Read the model definition and answer for the solid it produces. Units are mm, in the model's axes. Face numbers are marked on the shaded views. A direction names the side the tool comes from. Coordinates: 2 decimals unless noted, no trailing zeros. Loops run counter-clockwise (first coordinate to the right, second up) from the corner with the lowest first, then second, coordinate; pieces in that order, holes last.
from build123d import *

# Parameters (mm, degrees)
F1_DEPTH = 38.1
F2_R     = 3.175
F3_DEPTH = 25.4
F4_R     = 6.35
F6_DEPTH = 12.7
F7_R     = 12.7
F8_R     = 12.7


with BuildPart() as f1:
    # F0 (on Front) → F1 (new body)
    with BuildSketch(Plane.XZ):
        Polygon((19.5751538399, 3.9005766285), (19.3787731311, 22.9495643868), (-25.0712268689, 22.9495643868), (-25.0712268689, 18.1870643868), (-6.0212268689, 18.1870643868), (-6.0212268689, 8.6620643868), (-24.8748461601, 8.6620643868), (-24.8748461601, 3.9005766285), align=None)
    extrude(amount=-F1_DEPTH)

    # F2 (on face) → F3 (cut)
    with BuildSketch(Plane.XY.offset(22.9495643868)):
        with Locations((-15.5462268689, 28.575)):
            Circle(F2_R)
        with Locations((-15.5462268689, 9.525)):
            Circle(F2_R)
    extrude(amount=-F3_DEPTH, mode=Mode.SUBTRACT)

    # F4
    f4_edges = [f1.edges().sort_by_distance(p)[0] for p in [
        (-25.071227, 0, 20.568314),
        (-24.874846, 0, 6.281321),
        (-24.874846, 38.1, 6.281321),
        (-25.071227, 38.1, 20.568314),
    ]]
    fillet(f4_edges, radius=F4_R)

    # F5 (on face) → F6 (cut)
    with BuildSketch(Plane(origin=(19.613281335, 0, 0.2021981503), x_dir=(0, 1, 0), z_dir=(0.999946864, 0, 0.0103086986))):
        with BuildLine():
            Line((12.7, 13.2235750059), (25.4, 13.2235750059))
            ThreePointArc((25.4, 13.2235750059), (19.05, 19.5735750059), (12.7, 13.2235750059))
        make_face()
        with BuildLine():
            ThreePointArc((12.7, 13.2235750059), (19.05, 6.8735750059), (25.4, 13.2235750059))
            Line((25.4, 13.2235750059), (12.7, 13.2235750059))
        make_face()
    extrude(amount=-F6_DEPTH, mode=Mode.SUBTRACT)

    # F7
    f7_edges = [f1.edges().sort_by_distance(p)[0] for p in [
        (-6.021227, 0, 13.424564),
    ]]
    fillet(f7_edges, radius=F7_R)

    # F8
    f8_edges = [f1.edges().sort_by_distance(p)[0] for p in [
        (-6.021227, 38.1, 13.424564),
    ]]
    fillet(f8_edges, radius=F8_R)


solid = f1.part
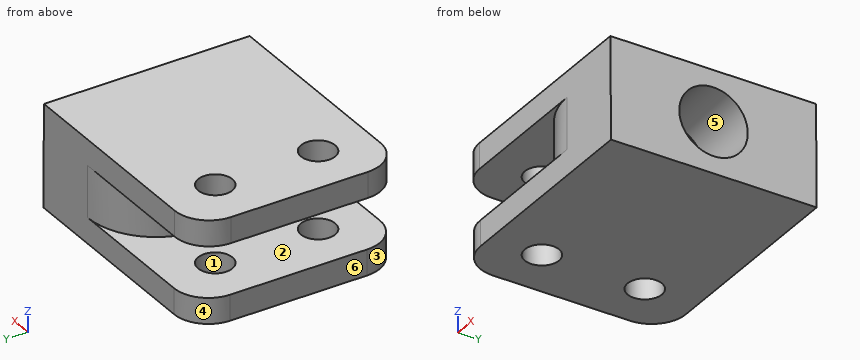
Item 1: A cutting plane is placed at A-A on x = -9. Determine the outline of the cut face in (y, z), then the cut area to 3 significant figures.
Numbers:
outline: (0, 3.9) - (38.1, 3.9) - (38.1, 8.66) - (0, 8.66) - close; (0, 18.19) - (38.1, 18.19) - (38.1, 22.95) - (0, 22.95) - close
area: 363 mm2
Item 2: Find the intervals of material crossed by line 1 along Z through (x, y) = (-22, 21.5); line 2 along Y through (x, z) = (15.5, 12.5); line 3 along Y through (x, z) = (13, 10), in increasing order.
Numbers:
line 1: z = 3.9 to 8.66, 18.19 to 22.95
line 2: y = 0 to 12.76, 25.34 to 38.1
line 3: y = 0 to 13.66, 24.44 to 38.1
Item 3: Which of the six approach directions +Z, -Z, +X, -X, +Y, -Y give full straight-line access (tool end or side, diameter ignored) to the marked faces 4, 5 and 6?
Numbers:
face 4: -Z, -X, +Y
face 5: none
face 6: -Z, -X, +Y, -Y
Item 4: A cutting plane is placed at B-B on y = 12. Determine the outline of the cut face in (x, z).
Numbers:
outline: (-25.07, 18.19) - (-17.53, 18.19) - (-17.53, 22.95) - (-25.07, 22.95) - close; (-24.87, 3.9) - (-17.53, 3.9) - (-17.53, 8.66) - (-24.87, 8.66) - close; (-13.56, 3.9) - (19.58, 3.9) - (19.38, 22.95) - (-13.56, 22.95) - (-13.56, 18.19) - (-6, 18.19) - (-6, 8.66) - (-13.56, 8.66) - close
Item 5: A cutting plane is placed at C-C on x = -13.5. Determine the outline of the cut face in (y, z), then the cut area to 3 significant figures.
Numbers:
outline: (0, 3.9) - (7.1, 3.9) - (7.1, 8.66) - (0, 8.66) - close; (0, 18.19) - (7.1, 18.19) - (7.1, 22.95) - (0, 22.95) - close; (11.95, 3.9) - (26.15, 3.9) - (26.15, 8.66) - (11.95, 8.66) - close; (11.95, 18.19) - (26.15, 18.19) - (26.15, 22.95) - (11.95, 22.95) - close; (31, 3.9) - (38.1, 3.9) - (38.1, 8.66) - (31, 8.66) - close; (31, 18.19) - (38.1, 18.19) - (38.1, 22.95) - (31, 22.95) - close
area: 270 mm2
Item 6: A cutting plane is placed at D-D on x = 2. Determine the outline of the cut face in (y, z).
Numbers:
outline: (0, 3.9) - (38.1, 3.9) - (38.1, 8.66) - (37.21, 8.66) - (37.21, 18.19) - (38.1, 18.19) - (38.1, 22.95) - (0, 22.95) - (0, 18.19) - (0.89, 18.19) - (0.89, 8.66) - (0, 8.66) - close
Item 7: Determine the mould class of the marked faces 1, 2 and 3 for opening direction Y: released by +Y, released by -Y, zero draft, split by the parting line, or undercut.
Numbers:
face 1: undercut
face 2: zero draft
face 3: released by -Y
Item 8: Given pin 1 (4 mm diameter, centred on x = -15.55, y = 9.52, fed in from +Z); pin 2 (3 mm diameter, centred on y = 18, z = 11.5, fed in from -X); pin 3 (5 mm diameter, centred on y = 25, z = 6.5, fed in from -X); pin 4 (8 mm diameter, centred on y = 23, z = 17, fed in from +X), each flat-ended and moving along its own axis, determine where each tip first touches the part or whether it passes through.
Numbers:
pin 1: passes through
pin 2: stops at x = -6.02
pin 3: stops at x = -24.87
pin 4: stops at x = 19.47
